from build123d import *

# Parameters (mm, degrees)
F0_W          = 76.319962422
F0_H          = 50.8
F1_DEPTH      = 6.35
F2_R          = 4.7045967167
F3_DEPTH      = 99
F3_DEPTH_BACK = 6.351


# Not quite as in the source:
# - an extrude ends at something that could not be found from the text; its depth is read off the source's solid
# - a feature names something its author has since deleted; it is built from what else it names


with BuildPart() as f1:
    # F0 (on Top) → F1 (new body)
    with BuildSketch(Plane.XY):
        with Locations((4.271581769, -3.4901092946)):
            Rectangle(F0_W, F0_H)
    extrude(amount=F1_DEPTH)

    # F2 (on face) → F3 (cut, two sides)
    with BuildSketch(Plane.XY.offset(6.35)) as f3_sk:
        with Locations((4.271581769, 9.693203494)):
            Circle(F2_R)
    extrude(amount=F3_DEPTH, mode=Mode.SUBTRACT)
    extrude(f3_sk.sketch, amount=-F3_DEPTH_BACK, mode=Mode.SUBTRACT)


solid = f1.part
Here's how the part is built. I have some questions about the finished solid (model axes, mm). Round coordinates to 2 decimals unless told otherwise and drop trailing zeros. Write each loop counter-clockwise with the first axis right and the second up, starting at its lowest first coordinate (ties: lowest second). Pieces come first, ordered by that corner, then holes.
1. Suppose I cut it at B-B (z = 4). List the corners of the cut face in (x, y) for me, and give its area (3 significant figures).
2. If we mould it in two halves opening along X, with no side actions, what happens to faces 1 (the flat face through (-33.888, -4, 3)), 2 (the flat face through (4, -28.89, 3)), 3 (the cylindrical face through (6.8, 13.66, 3.22))? For each: released by +X, released by -X, zero draft, split by the parting line, or undercut.
3. I need wall thicknesses on L1, parallel to X at y = 10, z = 2.75; L2, parallel to Y at x = 2.5, z = 2.25; L3, parallel to Y at x = 1, z = 3.5. Which ranges of each line are inside material? Lowest first, please.
4. Suppose I cut it at A-A (x = 7.5). List the corners of the cut face in (y, z) for me, and give its area (3 significant figures).
Answer sheet:
1. outline: (-33.89, -28.89) - (42.43, -28.89) - (42.43, 21.91) - (-33.89, 21.91) - close; hole circle Ø9.41 at (4.27, 9.69)
1. area: 3,810 mm2
2. face 1: released by -X
2. face 2: zero draft
2. face 3: undercut
3. L1: x = -33.89 to -0.42, 8.97 to 42.43
3. L2: y = -28.89 to 5.33, 14.05 to 21.91
3. L3: y = -28.89 to 6.31, 13.07 to 21.91
4. outline: (-28.89, 0) - (6.27, 0) - (6.27, 6.35) - (-28.89, 6.35) - close; (13.12, 0) - (21.91, 0) - (21.91, 6.35) - (13.12, 6.35) - close
4. area: 279 mm2
